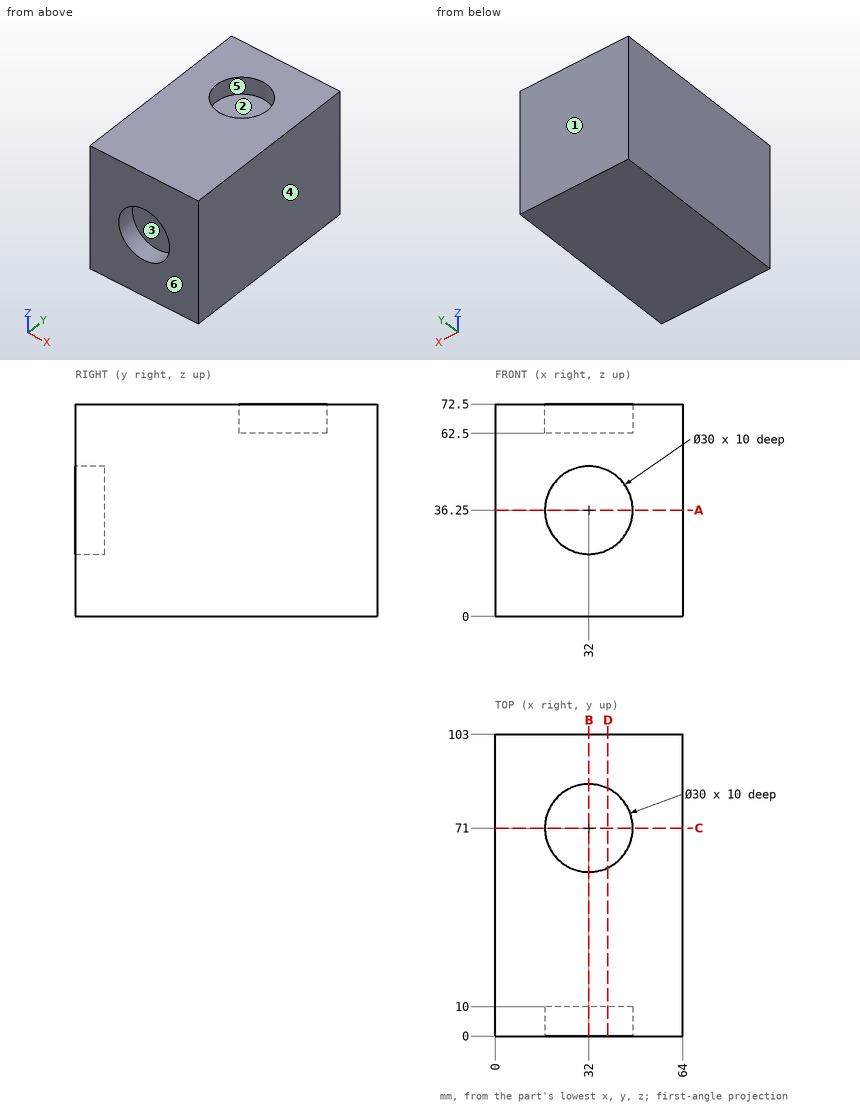
Answer from the drawing. Dimensions are ordinates in mm from the lowest x, y and z of the part. A direction names the side the tool comes from. Coordinates: 2 decimals unless noted, no trailing zeros. Write each loop counter-clockwise with the first axis right and the second up, starting at its lowest first coordinate (ties: lowest second). Pieces come first, ordered by that corner, then holes. Notation, with made-up numbers: (51.25, 49.5) - (80.25, 49.5) arc R14 ccw to (80.25, 57.5) - close; hole circle Ø11 at (60, -27). An arc over 180 degrees is marked (long way). One line per question, with ' | ' between items.
Q1. Find section C-C, the plane y = 71. Write down the section's boundary in (x, z), plus the area to 3 significant figures.
Result set:
outline: (0, 0) - (64, 0) - (64, 72.5) - (47, 72.5) - (47, 62.5) - (17, 62.5) - (17, 72.5) - (0, 72.5) - close | area: 4,340 mm^2
Q2. Determine the mould class of the marked faces 4, 5 and 6 for opening direction Y: +Y half, -Y half, draft (parallel to the pull), parting line (faces both ways), or undercut.
Result set:
face 4: draft | face 5: undercut | face 6: -Y half
Q3. Find section A-A, the plane z = 36.25. Write down the section's boundary in (x, y).
Result set:
outline: (0, 0) - (17, 0) - (17, 10) - (47, 10) - (47, 0) - (64, 0) - (64, 103) - (0, 103) - close
Q4. For the marked faces 1, 2 and 3, determine the directions among +Z, -Z, +X, -X, +Y, -Y from which every point of the face is accessible in a straight line to the end or side of a thin tool.
Result set:
face 1: +Z, -Z, +X, -X, +Y | face 2: +Z | face 3: -Y
Q5. Each of these flat-tipped pins is pushed along its axis until it touches: P1, Ø15, axis at x = 37, y = 67.5, coming from the +Z side; P2, Ø9, axis at x = 29, z = 35, coming from the -Y side. Where does it stop, or does it pass through?
Result set:
P1: z = 62.5 | P2: y = 10
Q6. Find section D-D, the plane x = 38.5. Write down the section's boundary in (y, z), plus the area to 3 significant figures.
Result set:
outline: (0, 0) - (103, 0) - (103, 72.5) - (84.52, 72.5) - (84.52, 62.5) - (57.48, 62.5) - (57.48, 72.5) - (0, 72.5) - (0, 49.77) - (10, 49.77) - (10, 22.73) - (0, 22.73) - close | area: 6,930 mm^2
Q7. Find section B-B, the plane x = 32. Write down the section's boundary in (y, z).
Result set:
outline: (0, 0) - (103, 0) - (103, 72.5) - (86, 72.5) - (86, 62.5) - (56, 62.5) - (56, 72.5) - (0, 72.5) - (0, 51.25) - (10, 51.25) - (10, 21.25) - (0, 21.25) - close
Q8. Consider L1, parallel to Y at x = 32, z = 67.5; L2, parallel to Z at x = 32, y = 81.5; L3, parallel to X at y = 4, z = 36. Determine where each line is inside the solid, lowest interval first. Write a range as [from, to].
Result set:
L1: [0, 56], [86, 103] | L2: [0, 62.5] | L3: [0, 17], [47, 64]
